```python
from build123d import *

# Parameters (mm, degrees)
F0_R     = 4
F0_R_2   = 1.5
F1_DEPTH = 15
F3_ANGLE = 180
F4_R     = 1.5
F5_DEPTH = 38.1


with BuildPart() as f1:
    # F0 (on Top) → F1 (new body)
    with BuildSketch(Plane.XY):
        Circle(F0_R)
        Circle(F0_R_2, mode=Mode.SUBTRACT)
    extrude(amount=F1_DEPTH)

    # F2 (on Front) → F3 (revolve, symmetric)
    with BuildSketch(Plane.XZ) as f3_sk:
        Polygon((-15, 13.998025), (0, 13.998025), (0, 17.998025), (-11, 17.998025), (-11, 40.998025), (0, 40.998025), (0, 43.998025), (-15, 43.998025), align=None)
    revolve(axis=Axis((0, 0, 21.028005), (0, 0, -1)), revolution_arc=F3_ANGLE / 2)
    revolve(f3_sk.sketch, axis=Axis((0, 0, 21.028005), (0, 0, 1)), revolution_arc=F3_ANGLE / 2)

    # F4 (on face) → F5 (cut)
    with BuildSketch(Plane.XY.offset(43.998025)):
        Circle(F4_R)
    extrude(amount=-F5_DEPTH, mode=Mode.SUBTRACT)


solid = f1.part
```
Design review of the part built by this model. Coordinates are the model's own, in mm. A direction names the side the tool comes from. Coordinates: 2 decimals unless noted, no trailing zeros. Write each loop counter-clockwise with the first axis right and the second up, starting at its lowest first coordinate (ties: lowest second). Pieces come first, ordered by that corner, then holes. Notation, with made-up numbers: M 33,55 L 39,55 A29 cw 39,86 Z; hole C 69,0 d6. An arc over 180 degrees is marked long. Answer as a JSON object with one key per item and string values.
Item 1: Wall thickness on probe 1 along Z at (x, y) = (-9.25, 5); probe 2 along Y at (x, z) = (0, 1.4): over which ranges is each line inside the solid? List them lowest first.
Outcome:
{"probe 1": "14 to 18, 41 to 44", "probe 2": "-4 to -1.5, 1.5 to 4"}
Item 2: Add section D-D, the plane x = 0.5. Give the boundary of the cut face in (y, z).
Outcome:
{"outline": "M -3.97,0 L -1.41,0 L -1.41,15 L -3.97,15 Z; M 1.41,0 L 3.97,0 L 3.97,15 L 1.41,15 Z"}
Item 3: Add section A-A, the plane y = 0. Give the boundary of the cut face in (x, z).
Outcome:
{"outline": "M -15,14 L -4,14 L -4,0 L -1.5,0 L -1.5,18 L -11,18 L -11,41 L -1.5,41 L -1.5,44 L -15,44 Z; M 1.5,0 L 4,0 L 4,15 L 1.5,15 Z"}
Item 4: Add section B-B, the plane x = -9.25. Give the boundary of the cut face in (y, z).
Outcome:
{"outline": "M -11.81,14 L 11.81,14 L 11.81,44 L -11.81,44 Z; hole M -5.95,18 L 5.95,18 L 5.95,41 L -5.95,41 Z"}
Item 5: Draft analysis for pull direction Y (two halves, no side actions). For faces 4 (the flat face through (0, -11.3, 29.2)), 5 (the flat face through (-4, 0, 40.998)), 6 (the cylindrical face through (-15, 0, 29)), state which applies: pulls with the +Y half, pulls with the -Y half, needs draft (parallel to the pull), parting line crosses it, or undercut.
Outcome:
{"face 4": "needs draft", "face 5": "undercut", "face 6": "parting line crosses it"}
Item 6: Add section C-C, the plane z = 5. Give the boundary of the cut face in (x, y).
Outcome:
{"outline": "C 0,0 d8; hole C 0,0 d3"}
Item 7: Insertion check: pin 1 Ø1.5 at (x, z) = (-3, 34.5) entering from -Y; pin 2 Ø4 at (x, y) = (-7.5, -8.5) entering from -Z; pin 3 Ø3 at (x, z) = (-9, 30) entering from +Y. Each pin has a flat end and moves straight along its axis. Give the tip position at first contact, or say it passes through.
Outcome:
{"pin 1": "y = -14.83", "pin 2": "z = 14", "pin 3": "y = 12.99"}
Item 8: Machinability: for faces 1 (the cylindrical face through (-11, 0, 30)), 2 (the flat face through (2, 0, 15)), 3 (the cylindrical face through (3.695, -1.532, 7.395)), which of the approach directions +Z, -Z, +X, -X, +Y, -Y give a long, thin tool a straight path to every point of the face, cutting with its end or side? Answer none if there is none.
Outcome:
{"face 1": "+X", "face 2": "+Z, +X, +Y, -Y", "face 3": "-Z"}
